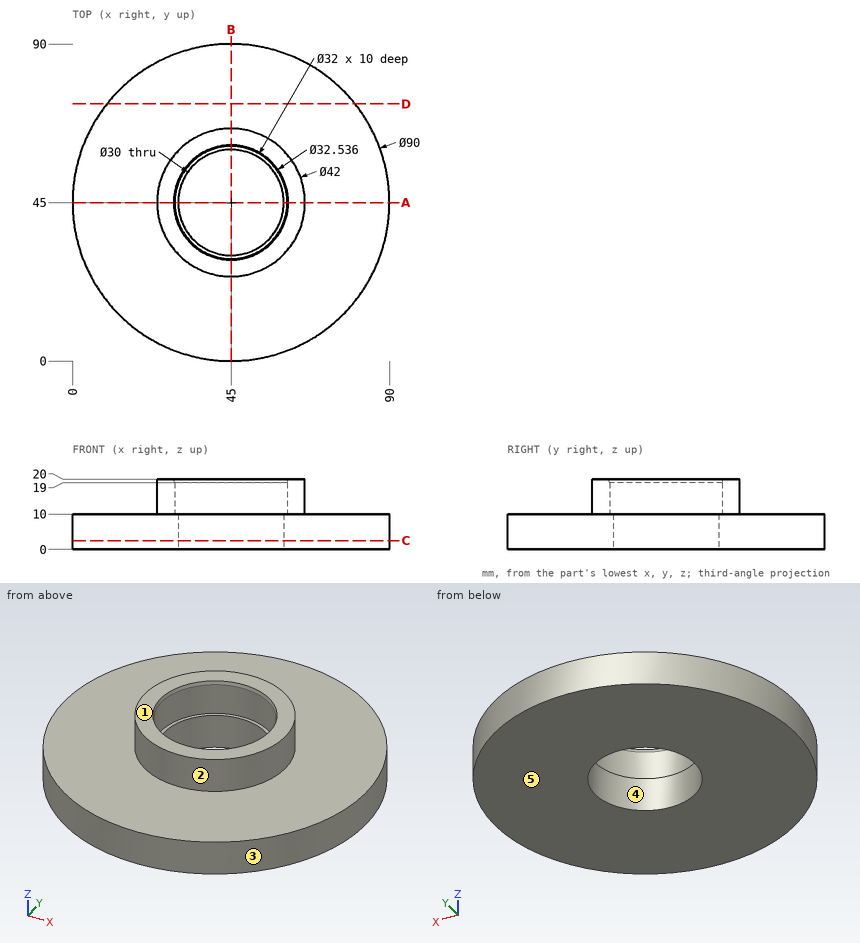
Geometry: see drawing. Coordinates: mm, zero at the bounding-box minimum. A direction names the side the tool comes from. Round coordinates to 2 decimals unless told otherwise and drop trailing zeros. Order: outer loops, then holes, each group sorted by start corner. A loop starts at its lowest first (then second) coordinate and runs counter-clockwise, first axis right, second up. Notation, with made-up numbers: (51, -0.75) -> (105, -0.75) arc R19 ccw to (105, 33.25) -> close; hole circle Ø10 at (-29, -15). An arc over 180 degrees is marked (long way). Answer as CSV lines item,"result".
Item 1: Section C-C, the plane z = 2.5. Return loops of the section in (x, y), plus the area to 3 significant figures.
A:
outline,"circle Ø90 at (45, 45); hole circle Ø30 at (45, 45)"
area,"5,650 mm²"
Item 2: Reachability of the marked faces 1 and 2 from +Z, -Z, +X, -X, +Y, -Y: full face, straight path, thin tool, end or side. Return the list, or none.
A:
face 1,"+Z, +X, -X, +Y, -Y"
face 2,"+Z"
Item 3: Line query: L1, parallel to Y at x = 45, z = 6; L2, parallel to Y at x = 45, z = 14.5; L3, parallel to Z at x = 10.5, y = 53.5. Output: solid intervals per line, ascending.
A:
L1,"0 to 30, 60 to 90"
L2,"24 to 29, 61 to 66"
L3,"0 to 10"
Item 4: Section A-A, the plane y = 45. Return loops of the section in (x, z), plus the area to 3 significant figures.
A:
outline,"(0, 0) -> (30, 0) -> (30, 10) -> (29, 10) -> (29, 19) -> (28.73, 20) -> (24, 20) -> (24, 10) -> (0, 10) -> close; (60, 0) -> (90, 0) -> (90, 10) -> (66, 10) -> (66, 20) -> (61.27, 20) -> (61, 19) -> (61, 10) -> (60, 10) -> close"
area,"700 mm²"
Item 5: Section D-D, the plane y = 73. Return loops of the section in (x, z).
A:
outline,"(9.77, 0) -> (80.23, 0) -> (80.23, 10) -> (9.77, 10) -> close"
Item 6: Pull-direction query (X, two-part tool) for the marked faces 3, 4 and 5; classes: pulls with the +X half, pulls with the -X half, needs draft (parallel to the pull), parting line crosses it, or undercut.
A:
face 3,"parting line crosses it"
face 4,"undercut"
face 5,"needs draft"
Item 7: Pin query (flat end, axial travel): pin 1 Ø1.5 at (y, z) = (10, 4) entering from +X; pin 2 Ø19 at (x, y) = (45, 45) entering from -Z; pin 3 Ø5 at (x, z) = (69.5, 3.5) entering from +Y; pin 4 Ø2 at (y, z) = (31.5, 15) entering from -X. Return the tip coordinate at first contact, or that it passes through.
A:
pin 1,"x = 74.19"
pin 2,"through"
pin 3,"y = 84.26"
pin 4,"x = 28.13"
